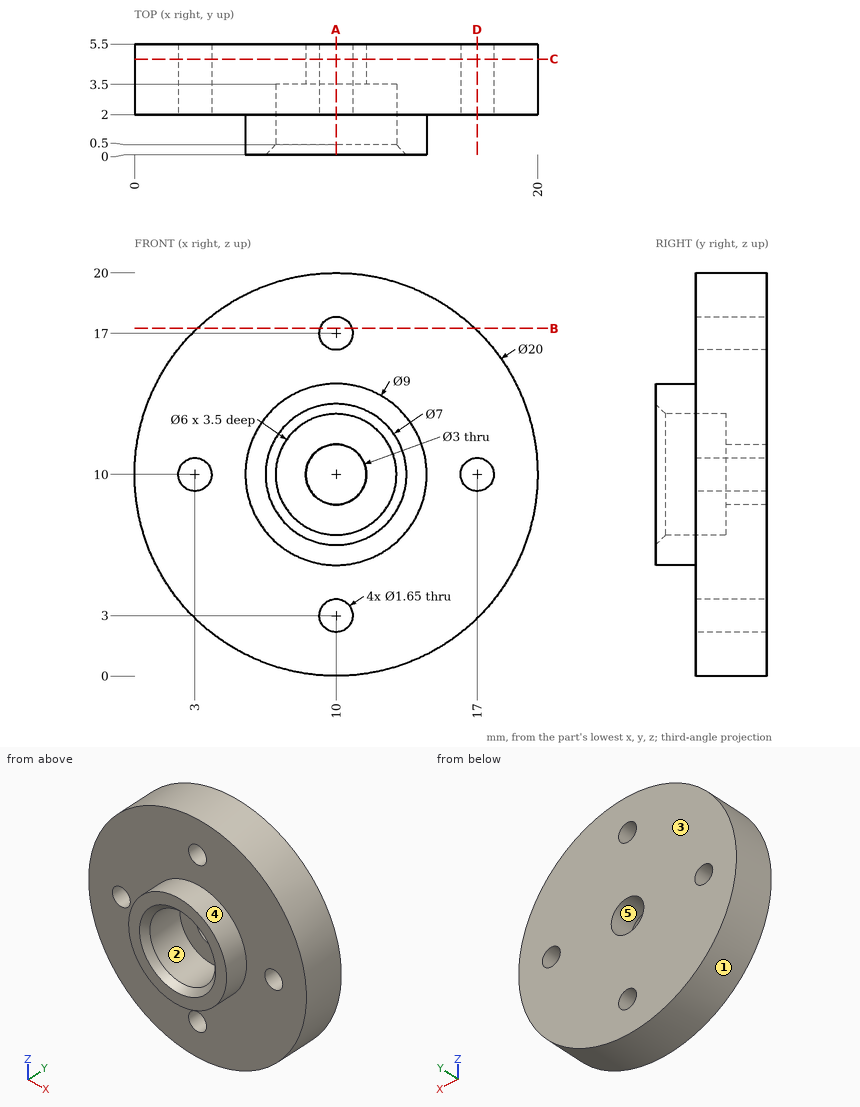
Answer from the drawing. Dimensions are ordinates in mm from the lowest x, y and z of the part. A direction names the side the tool comes from. Give positions to 0.01 mm unless a question says otherwise; leave off trailing zeros. Loops run counter-clockwise (first coordinate to the right, second up) from the corner with the lowest first, then second, coordinate; pieces in that order, holes last.
Item 1: The part is cut by section A-A (x = 10). Write down the section's boundary in (y, z) (3 decimals), and give its area (3 significant figures).
Item 2: Each of these flat-tipped pins is pushed along its axis until it touches: pin 1 Ø1 at (x, z) = (8, 6) entering from -Y; pin 2 Ø1.9 at (x, z) = (3, 10) entering from -Y; pin 3 Ø2 at (x, y) = (11.5, 4.5) entering from +Z; pin 4 Ø3 at (y, z) = (5, 16) entering from +X. Where does it stop, or does it pass through?
Item 3: For the marked faces 4 and 5, determine the directions among +Z, -Z, +X, -X, +Y, -Y from which every point of the face is accessible in a straight line to the end or side of a thin tool.
Item 4: Find the intervals of material crossed by line 1 along X through (y, z) = (4, 10) (3 decimals); line 2 along X through (y, z) = (1.5, 10); line 3 along Y through (x, z) = (14, 15.5), in increasing order.
Item 5: The mould has two halves that part along Z. Classify the marked faces 1, 2 and 3: released by +Z, released by -Z, zero draft, split by the parting line, or undercut.
Item 6: The part is cut by section B-B (z = 17.25). Write down the section's boundary in (x, y), and give its area (3 significant figures).
Item 7: The part is cut by section D-D (x = 17). Write down the section's boundary in (y, z) (3 decimals).
Item 8: The part is cut by section C-C (y = 4.75). Write down the section's boundary in (x, z) (3 decimals).
Taken from the geometry:
1. outline: (0, 5.5) - (2, 5.5) - (2, 3.825) - (5.5, 3.825) - (5.5, 8.5) - (3.5, 8.5) - (3.5, 7) - (0.5, 7) - (0, 6.5) - close; (0, 13.5) - (0.5, 13) - (3.5, 13) - (3.5, 11.5) - (5.5, 11.5) - (5.5, 16.175) - (2, 16.175) - (2, 14.5) - (0, 14.5) - close; (2, 0) - (5.5, 0) - (5.5, 2.175) - (2, 2.175) - close; (2, 17.825) - (5.5, 17.825) - (5.5, 20) - (2, 20) - close
1. area: 49.2 mm2
2. pin 1: stops at y = 0
2. pin 2: stops at y = 2
2. pin 3: stops at z = 19.99
2. pin 4: stops at x = 18.93
3. face 4: -Y
3. face 5: +Y, -Y
4. line 1: x = 0 to 2.175, 3.825 to 8.5, 11.5 to 16.175, 17.825 to 20
4. line 2: x = 5.5 to 7, 13 to 14.5
4. line 3: y = 2 to 5.5
5. face 1: split by the parting line
5. face 2: undercut
5. face 3: zero draft
6. outline: (3.11, 2) - (9.21, 2) - (9.21, 5.5) - (3.11, 5.5) - close; (10.79, 2) - (16.89, 2) - (16.89, 5.5) - (10.79, 5.5) - close
6. area: 42.7 mm2
7. outline: (2, 2.859) - (5.5, 2.859) - (5.5, 9.175) - (2, 9.175) - close; (2, 10.825) - (5.5, 10.825) - (5.5, 17.141) - (2, 17.141) - close
8. outline: circle Ø20 at (10, 10); hole circle Ø1.65 at (3, 10); hole circle Ø3 at (10, 10); hole circle Ø1.65 at (10, 3); hole circle Ø1.65 at (10, 17); hole circle Ø1.65 at (17, 10)
